The listing builds one solid part. Answer for the finished solid, in the listing's coordinates (mm). A direction names the side the tool comes from. Coordinates: 2 decimals unless noted, no trailing zeros. Write each loop counter-clockwise with the first axis right and the second up, starting at its lowest first coordinate (ties: lowest second). Pieces come first, ordered by that corner, then holes.
(1) Which of the six approach directions +Z, -Z, +X, -X, +Y, -Y give full straight-line access (tool end or side, diameter ignored) to faces 1 (the flat face through (24.1, 1, -10)), 2 (the flat face through (24, 2, -19))?
(2) For a pull along Z with two mould halves and no side action, classify faces 3 (the flat face through (22.594, 1.014, -2.347)), 4 (the flat face through (43, 1, -30)), 5 (the cylindrical face through (3, 0.99, -5.46)), 6 (the cylindrical face through (41.128, 0.986, -10.386)) as +Z half, -Z half, draft (parallel to the pull), parting line (faces both ways), or undercut.
(3) The part is cut by section A-A on x = 41.5. Determine the outline of the cut face in (y, z), plus the area to 3 significant figures.
(4) Given P1, Ø1.1, axis at y = 1.5, z = -28.5, coming from the +X side; P2, Ø1.5, axis at x = -4.5, z = -8.5, coming from the +Y side; P3, Ø0.5, axis at y = 1, z = -28.5, coming from the +X side; P4, Ø0.8, axis at y = 1, z = -1.5, coming from the +X side, each flat-ended and moving along its own axis, determine where each tip first touches the part or whether it passes through.
(5) The part is cut by section D-D on z = -7.5. Determine the outline of the cut face in (x, y), plus the area to 3 significant figures.
(6) The part is cut by section C-C on y = 1.15. Give the number of separate pieces and of enclosed holes in the cut face, plus the area to 3 significant figures.
(7) The part is cut by section B-B on z = -17.5. Determine the outline of the cut face in (x, y), plus the area to 3 significant figures.
(8) Straight lines are drawn through the part: line 1 (X direction, y = 1.35, z = -15); line 2 (X direction, y = 1.8, z = -14.5); line 3 (X direction, y = 1.75, z = -23). For each, find the intervals that lie inside material, in ascending order.
from build123d import *

# Parameters (mm, degrees)
SKETCH1_R           = 10
SKETCH1_R_2         = 1
BOSS_EXTRUDE1_DEPTH = 2
SKETCH2_W           = 2
SKETCH2_H           = 3
CUT_EXTRUDE1_DEPTH  = 72.617037079
FILLET1_START       = -1
FILLET1_DEPTH       = 4
FILLET1_2_DEPTH     = 2
CUT_EXTRUDE2_DEPTH  = 72.617037079
FILLET2_R           = 1


with BuildPart() as part:
    # Sketch1 → Boss-Extrude1 (new body)
    with BuildSketch(Plane(origin=(0, 0, 0), x_dir=(1, 0, 0), z_dir=(0, 1, 0))):
        with BuildLine():
            Line((0, 0), (50, 0))
            ThreePointArc((50, 0), (65, 15), (50, 30))
            Line((50, 30), (0, 30))
            ThreePointArc((0, 30), (-15, 15), (0, 0))
        make_face()
        with Locations(Location((0, 15, 0), (0, 0, 270))):
            Circle(SKETCH1_R, mode=Mode.SUBTRACT)
        with Locations(Location((50, 15, 0), (0, 0, 270))):
            Circle(SKETCH1_R, mode=Mode.SUBTRACT)
        with Locations(Location((25, 15, 0), (0, 0, 270))):
            Circle(SKETCH1_R_2, mode=Mode.SUBTRACT)
    extrude(amount=BOSS_EXTRUDE1_DEPTH)

    # Sketch2 → Cut-Extrude1 (cut, through all)
    with BuildSketch(Plane(origin=(0, 2, 0), x_dir=(1, 0, 0), z_dir=(0, 1, 0))):
        with Locations((17, 28.5)):
            Rectangle(SKETCH2_W, SKETCH2_H)
        with Locations((33, 28.5)):
            Rectangle(SKETCH2_W, SKETCH2_H)
        with Locations((17, 1.5)):
            Rectangle(SKETCH2_W, SKETCH2_H)
        with Locations((33, 1.5)):
            Rectangle(SKETCH2_W, SKETCH2_H)
    extrude(amount=-CUT_EXTRUDE1_DEPTH, mode=Mode.SUBTRACT)

    # Fillet1: read off the stored shape, not the designer's step
    # Fillet1 outline → Fillet1 (cut)
    with BuildSketch(Plane(origin=(0, 0, 0), x_dir=(1, 0, 0), z_dir=(0, 1, 0)).offset(FILLET1_START)):
        with BuildLine():
            ThreePointArc((35, 0), (34.292893219, 0.292893219), (34, 1))
            Line((34, 1), (34, 0))
            Line((34, 0), (35, 0))
        make_face()
        with BuildLine():
            ThreePointArc((32, 1), (31.707106781, 0.292893219), (31, 0))
            Line((31, 0), (32, 0))
            Line((32, 0), (32, 1))
        make_face()
        with BuildLine():
            ThreePointArc((19, 0), (18.292893219, 0.292893219), (18, 1))
            Line((18, 1), (18, 0))
            Line((18, 0), (19, 0))
        make_face()
        with BuildLine():
            ThreePointArc((16, 1), (15.707106781, 0.292893219), (15, 0))
            Line((15, 0), (16, 0))
            Line((16, 0), (16, 1))
        make_face()
        with BuildLine():
            ThreePointArc((15, 30), (15.707106781, 29.707106781), (16, 29))
            Line((16, 29), (16, 30))
            Line((16, 30), (15, 30))
        make_face()
        with BuildLine():
            ThreePointArc((18, 29), (18.292893219, 29.707106781), (19, 30))
            Line((19, 30), (18, 30))
            Line((18, 30), (18, 29))
        make_face()
        with BuildLine():
            ThreePointArc((31, 30), (31.707106781, 29.707106781), (32, 29))
            Line((32, 29), (32, 30))
            Line((32, 30), (31, 30))
        make_face()
        with BuildLine():
            ThreePointArc((34, 29), (34.292893219, 29.707106781), (35, 30))
            Line((35, 30), (34, 30))
            Line((34, 30), (34, 29))
        make_face()
    extrude(amount=FILLET1_DEPTH, mode=Mode.SUBTRACT)

    # Fillet1 2 outline → Fillet1 2 (add)
    with BuildSketch(Plane(origin=(0, 0, 0), x_dir=(1, 0, 0), z_dir=(0, 1, 0))):
        with BuildLine():
            Line((34, 3), (33, 3))
            ThreePointArc((33, 3), (33.707106781, 2.707106781), (34, 2))
            Line((34, 2), (34, 3))
        make_face()
        with BuildLine():
            Line((32, 3), (32, 2))
            ThreePointArc((32, 2), (32.292893219, 2.707106781), (33, 3))
            Line((33, 3), (32, 3))
        make_face()
        with BuildLine():
            Line((18, 3), (17, 3))
            ThreePointArc((17, 3), (17.707106781, 2.707106781), (18, 2))
            Line((18, 2), (18, 3))
        make_face()
        with BuildLine():
            Line((16, 3), (16, 2))
            ThreePointArc((16, 2), (16.292893219, 2.707106781), (17, 3))
            Line((17, 3), (16, 3))
        make_face()
        with BuildLine():
            Line((16, 27), (17, 27))
            ThreePointArc((17, 27), (16.292893219, 27.292893219), (16, 28))
            Line((16, 28), (16, 27))
        make_face()
        with BuildLine():
            Line((18, 27), (18, 28))
            ThreePointArc((18, 28), (17.707106781, 27.292893219), (17, 27))
            Line((17, 27), (18, 27))
        make_face()
        with BuildLine():
            Line((32, 27), (33, 27))
            ThreePointArc((33, 27), (32.292893219, 27.292893219), (32, 28))
            Line((32, 28), (32, 27))
        make_face()
        with BuildLine():
            Line((34, 27), (34, 28))
            ThreePointArc((34, 28), (33.707106781, 27.292893219), (33, 27))
            Line((33, 27), (34, 27))
        make_face()
    extrude(amount=FILLET1_2_DEPTH)

    # Sketch3 → Cut-Extrude2 (cut, through all)
    with BuildSketch(Plane(origin=(0, 2, 0), x_dir=(1, 0, 0), z_dir=(0, 1, 0))):
        Polygon((24.1, 14.564110106), (25.9, 14.564110106), (25.9, 4.564110106), (29, 0), (21, 0), (24.1, 4.564110106), align=None)
    extrude(amount=-CUT_EXTRUDE2_DEPTH, mode=Mode.SUBTRACT)

    # Fillet2
    fillet2_edges = [part.edges().sort_by_distance(p)[0] for p in [
        (24.1, 1, -4.564110106),
        (24.1, 1, -14.564110106),
        (25.9, 1, -14.564110106),
        (25.9, 1, -4.564110106),
        (29, 1, 0),
        (21, 1, 0),
    ]]
    fillet(fillet2_edges, radius=FILLET2_R)


solid = part.part
Model answer:
1. face 1: +Z, +Y, -Y
1. face 2: +Z, -Z, +X, -X, +Y
2. face 3: +Z half
2. face 4: -Z half
2. face 5: undercut
2. face 6: undercut
3. outline: (0, -30) - (2, -30) - (2, -20.27) - (0, -20.27) - close; (0, -9.73) - (2, -9.73) - (2, 0) - (0, 0) - close
3. area: 38.9 mm2
4. P1: stops at x = 57.57
4. P2: passes through
4. P3: stops at x = 57.03
4. P4: stops at x = 57.31
5. outline: (-12.99, 0) - (-6.61, 0) - (-6.61, 2) - (-12.99, 2) - close; (6.61, 0) - (24.1, 0) - (24.1, 2) - (6.61, 2) - close; (25.9, 0) - (43.39, 0) - (43.39, 2) - (25.9, 2) - close; (56.61, 0) - (62.99, 0) - (62.99, 2) - (56.61, 2) - close
5. area: 95.4 mm2
6. separate pieces: 1
6. enclosed holes: 2
6. area: 1,510 mm2
7. outline: (-14.79, 0) - (-9.68, 0) - (-9.68, 2) - (-14.79, 2) - close; (9.68, 0) - (40.32, 0) - (40.32, 2) - (9.68, 2) - close; (59.68, 0) - (64.79, 0) - (64.79, 2) - (59.68, 2) - close
7. area: 81.7 mm2
8. line 1: x = -15 to -10, 10 to 24, 26 to 40, 60 to 65
8. line 2: x = -14.99 to -9.99, 9.99 to 24.09, 25.91 to 40.01, 59.99 to 64.99
8. line 3: x = -12.69 to -6, 6 to 44, 56 to 62.69
